Input: part model. Units: mm. Frame: model coordinates. Face numbers are marked on the shaded views. A direction names the side the tool comes from. Round coordinates to 2 decimals unless told otherwise and drop trailing zeros. Loops run counter-clockwise (first coordinate to the right, second up) from the corner with the lowest first, then second, coordinate; pieces in that order, holes last. Notation, with made-up numbers: (-2, 51) - (39, 51) arc R32 ccw to (39, 84) - close; hole circle Ø3 at (-28.5, 1.5). An arc over 180 degrees is marked (long way). One line per question, with ' | ' between items. Start each with the question number.
Item 1: First-contact query: pin 1 (1.7 mm diameter, centred on x = -17.98, z = 0, fed in from +Y); pin 2 (1 mm diameter, centred on x = -35, y = -11.5, fed in from -Z); pin 3 (3 mm diameter, centred on x = 33, y = -4, fed in from -Z). Flat tips, straight axial feed; report the tip coordinate or a pass-through.
Item 2: Set-up query: the marked faces 1 and 2. Return all of +Z, -Z, +X, -X, +Y, -Y with unobstructed straight access to the full face (end or side cutting, diameter ignored); none if empty.
Item 3: Section B-B, the plane x = 41.5. Return loops of the section in (y, z), plus the area to 3 significant figures.
Item 4: Draft query along Z for the marked faces 3, 4 and 5. Return one class per face: pulls with the +Z half, pulls with the -Z half, needs draft (parallel to the pull), parting line crosses it, or undercut.
Item 5: Section D-D, the plane x = -42.5. Return loops of the section in (y, z), plus the area to 3 significant figures.
Item 6: Section C-C, the plane z = 41. Return loops of the section in (x, y), plus the area to 3 significant figures.
Item 7: Section A-A, the plane y = -2. Return loops of the section in (x, z) (3 decimals), plus the area to 3 significant figures.
Item 8: Material intervals for line 1 along X through (y, z) = (-1.5, 0); line 2 along Z through (x, y) = (15.5, -11.25); line 3 along Z through (x, y) = (3, -1.5), sorted ascending.
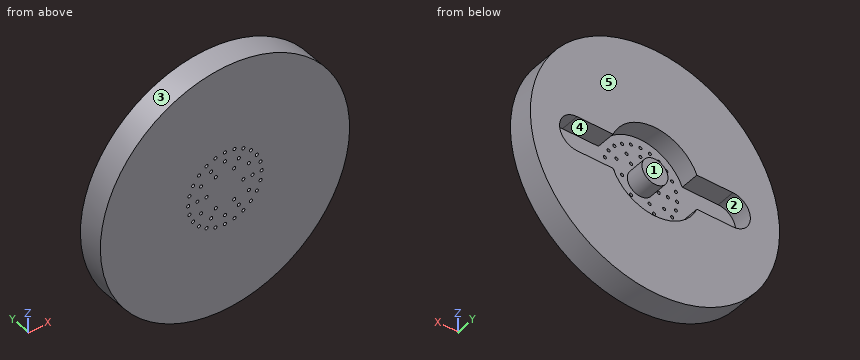
```python
from build123d import *

# Parameters (mm, degrees)
SKETCH1_R                       = 60.96
BILLET_DEPTH                    = 12.7
SKETCH4_R                       = 0.7493
FIRST_KEROSENE_OUTLET_DEPTH     = 88.140881336
PRIMARY_HOLES_COUNT             = 6
SECOND_START                    = -12.7
SECOND_RING_OUTLINE_R           = 0.7493
SECOND_RING_DEPTH               = 12.7
THIRD_START                     = -12.7
THIRD_RING_OUTLINE_R            = 0.7493
THIRD_RING_DEPTH                = 12.7
KEROSENE_WELL_DEPTH             = 9.3218
SKETCH17_R                      = 6.35
BOSS_EXTRUDE1_DEPTH             = 2.54
BOSS_EXTRUDE1_DIRECTION_2_REACH = 89.141
SKETCH19_R                      = 6.35
LOX_TOWER_DEPTH                 = 2.54


# Read off the part's stored shape, not the designer's step: Second ring, Third Ring
with BuildPart() as part:
    # Sketch1 → Billet (new body)
    with BuildSketch(Plane(origin=(0, 0, 0), x_dir=(1, 0, 0), z_dir=(0, 1, 0))):
        with Locations(Location((0, 0, 0), (0, 0, 270))):
            Circle(SKETCH1_R)
    extrude(amount=-BILLET_DEPTH)

    # Sketch4 → First Kerosene Outlet (cut, symmetric)
    with BuildSketch(Plane(origin=(0, -12.7, 0), x_dir=(1, 0, 0), z_dir=(0, 1, 0))):
        with Locations(Location((8.9916, 0, 0), (0, 0, 270))):
            Circle(SKETCH4_R)
        with Locations(Location((13.4874, 0, 0), (0, 0, 270))):
            Circle(SKETCH4_R)
        with Locations(Location((17.9832, 0, 0), (0, 0, 270))):
            Circle(SKETCH4_R)
    first_kerosene_outlet = extrude(amount=FIRST_KEROSENE_OUTLET_DEPTH, both=True, mode=Mode.SUBTRACT)

    # Primary Holes: First Kerosene Outlet ×6 about axis
    primary_holes_axis = Axis((0, 0, 0), (0, 1, 0))
    for i in range(1, PRIMARY_HOLES_COUNT):
        add(first_kerosene_outlet.rotate(primary_holes_axis, i * 360 / PRIMARY_HOLES_COUNT), mode=Mode.SUBTRACT)

    # Second ring outline → Second ring (cut)
    with BuildSketch(Plane(origin=(0, 0, 0), x_dir=(1, 0, 0), z_dir=(0, 1, 0)).offset(SECOND_START)):
        with Locations((11.680431031, 6.7437)):
            Circle(SECOND_RING_OUTLINE_R)
        with Locations((0, 13.4874)):
            Circle(SECOND_RING_OUTLINE_R)
        with Locations((-11.680431031, 6.7437)):
            Circle(SECOND_RING_OUTLINE_R)
        with Locations((-11.680431031, -6.7437)):
            Circle(SECOND_RING_OUTLINE_R)
        with Locations((0, -13.4874)):
            Circle(SECOND_RING_OUTLINE_R)
        with Locations((11.680431031, -6.7437)):
            Circle(SECOND_RING_OUTLINE_R)
    extrude(amount=SECOND_RING_DEPTH, mode=Mode.SUBTRACT)

    # Third Ring outline → Third Ring (cut)
    with BuildSketch(Plane(origin=(0, 0, 0), x_dir=(1, 0, 0), z_dir=(0, 1, 0)).offset(THIRD_START)):
        with Locations((17.370437319, 4.654394652)):
            Circle(THIRD_RING_OUTLINE_R)
        with Locations((15.573908041, 8.9916)):
            Circle(THIRD_RING_OUTLINE_R)
        with Locations((12.716042667, 12.716042667)):
            Circle(THIRD_RING_OUTLINE_R)
        with Locations((4.654394652, 17.370437319)):
            Circle(THIRD_RING_OUTLINE_R)
        with Locations((0, 17.9832)):
            Circle(THIRD_RING_OUTLINE_R)
        with Locations((-4.654394652, 17.370437319)):
            Circle(THIRD_RING_OUTLINE_R)
        with Locations((-12.716042667, 12.716042667)):
            Circle(THIRD_RING_OUTLINE_R)
        with Locations((-15.573908041, 8.9916)):
            Circle(THIRD_RING_OUTLINE_R)
        with Locations((-17.370437319, 4.654394652)):
            Circle(THIRD_RING_OUTLINE_R)
        with Locations((-17.370437319, -4.654394652)):
            Circle(THIRD_RING_OUTLINE_R)
        with Locations((-15.573908041, -8.9916)):
            Circle(THIRD_RING_OUTLINE_R)
        with Locations((-12.716042667, -12.716042667)):
            Circle(THIRD_RING_OUTLINE_R)
        with Locations((-4.654394652, -17.370437319)):
            Circle(THIRD_RING_OUTLINE_R)
        with Locations((0, -17.9832)):
            Circle(THIRD_RING_OUTLINE_R)
        with Locations((4.654394652, -17.370437319)):
            Circle(THIRD_RING_OUTLINE_R)
        with Locations((12.716042667, -12.716042667)):
            Circle(THIRD_RING_OUTLINE_R)
        with Locations((15.573908041, -8.9916)):
            Circle(THIRD_RING_OUTLINE_R)
        with Locations((17.370437319, -4.654394652)):
            Circle(THIRD_RING_OUTLINE_R)
    extrude(amount=THIRD_RING_DEPTH, mode=Mode.SUBTRACT)

    # Sketch18 → Kerosene Well (cut)
    with BuildSketch(Plane(origin=(0, 0, 0), x_dir=(1, 0, 0), z_dir=(0, 1, 0))):
        with BuildLine():
            Line((-38.1, 8.57504), (-20.504129194, 8.57504))
            ThreePointArc((-20.504129194, 8.57504), (0, 22.225), (20.504129194, 8.57504))
            Line((20.504129194, 8.57504), (38.1, 8.57504))
            ThreePointArc((38.1, 8.57504), (46.67504, 0), (38.1, -8.57504))
            Line((38.1, -8.57504), (20.504129194, -8.57504))
            ThreePointArc((20.504129194, -8.57504), (0, -22.225), (-20.504129194, -8.57504))
            Line((-20.504129194, -8.57504), (-38.1, -8.57504))
            ThreePointArc((-38.1, -8.57504), (-46.67504, 0), (-38.1, 8.57504))
        make_face()
    extrude(amount=-KEROSENE_WELL_DEPTH, mode=Mode.SUBTRACT)

    # Sketch17 → Boss-Extrude1 (add)
    with BuildSketch(Plane(origin=(0, 0, 0), x_dir=(1, 0, 0), z_dir=(0, 1, 0))):
        with Locations(Location((0, 0, 0), (0, 0, 270))):
            Circle(SKETCH17_R)
    extrude(amount=BOSS_EXTRUDE1_DEPTH)

    # Sketch17 → Boss-Extrude1 direction 2 (add, up to next)
    with BuildSketch(Plane(origin=(0, 0, 0), x_dir=(1, 0, 0), z_dir=(0, 1, 0)), mode=Mode.PRIVATE) as boss_extrude1_direction_2_sk1:
        with Locations(Location((0, 0, 0), (0, 0, 270))):
            Circle(SKETCH17_R)
    boss_extrude1_direction_2_tool1 = extrude(boss_extrude1_direction_2_sk1.sketch, amount=-BOSS_EXTRUDE1_DIRECTION_2_REACH, mode=Mode.PRIVATE) - part.part
    add(boss_extrude1_direction_2_tool1.solids().sort_by_distance((0, 0, 0))[0])

    # Sketch19 → Lox Tower (cut)
    with BuildSketch(Plane(origin=(0, 2.54, 0), x_dir=(1, 0, 0), z_dir=(0, 1, 0))):
        with Locations(Location((0, 0, 0), (0, 0, 270))):
            Circle(SKETCH19_R)
    extrude(amount=-LOX_TOWER_DEPTH, mode=Mode.SUBTRACT)


solid = part.part
```
Return value:
1) pin 1: y = -9.32 | pin 2: z = -50.26 | pin 3: z = -52.19
2) face 1: +Z, -Z, +X, -X, +Y | face 2: +Y
3) outline: (-12.7, -44.65) - (0, -44.65) - (0, -7.87) - (-9.32, -7.87) - (-9.32, 7.87) - (0, 7.87) - (0, 44.65) - (-12.7, 44.65) - close | area: 987 mm2
4) face 3: parting line crosses it | face 4: undercut | face 5: needs draft
5) outline: (-12.7, -43.7) - (0, -43.7) - (0, -7.36) - (-9.32, -7.36) - (-9.32, 7.36) - (0, 7.36) - (0, 43.7) - (-12.7, 43.7) - close | area: 973 mm2
6) outline: (-45.11, -12.7) - (45.11, -12.7) - (45.11, 0) - (-45.11, 0) - close | area: 1,150 mm2
7) outline: circle Ø121.92 at (0, 0); circle Ø12.7 at (0, 0); hole (-38.1, -8.575) - (-20.504, -8.575) arc R22.225 ccw to (20.504, -8.575) - (38.1, -8.575) arc R8.575 ccw to (38.1, 8.575) - (20.504, 8.575) arc R22.225 ccw to (-20.504, 8.575) - (-38.1, 8.575) arc R8.575 ccw to start | area: 9,450 mm2
8) line 1: -60.96 to -46.68, -6.35 to 6.35, 46.68 to 60.96 | line 2: -58.96 to -9.74, -8.25 to 8.25, 9.74 to 58.96 | line 3: -60.89 to -22.02, -5.6 to 5.6, 22.02 to 60.89
